Could you check a few things on this drawing? It's one solid part, dimensions in mm from its lowest x, y, z. Coordinates: 2 decimals unless noted, no trailing zeros. Order: outer loops, then holes, each group sorted by start corner. A loop starts at its lowest first (then second) coordinate and runs counter-clockwise, first axis right, second up. Notation, with made-up numbers: M 21,20 L 51,20 A24 cw 51,41 Z; hole C 79,42.5 d8. An arc over 180 degrees is marked long. Write item = value, one per line. Start each with the question number.
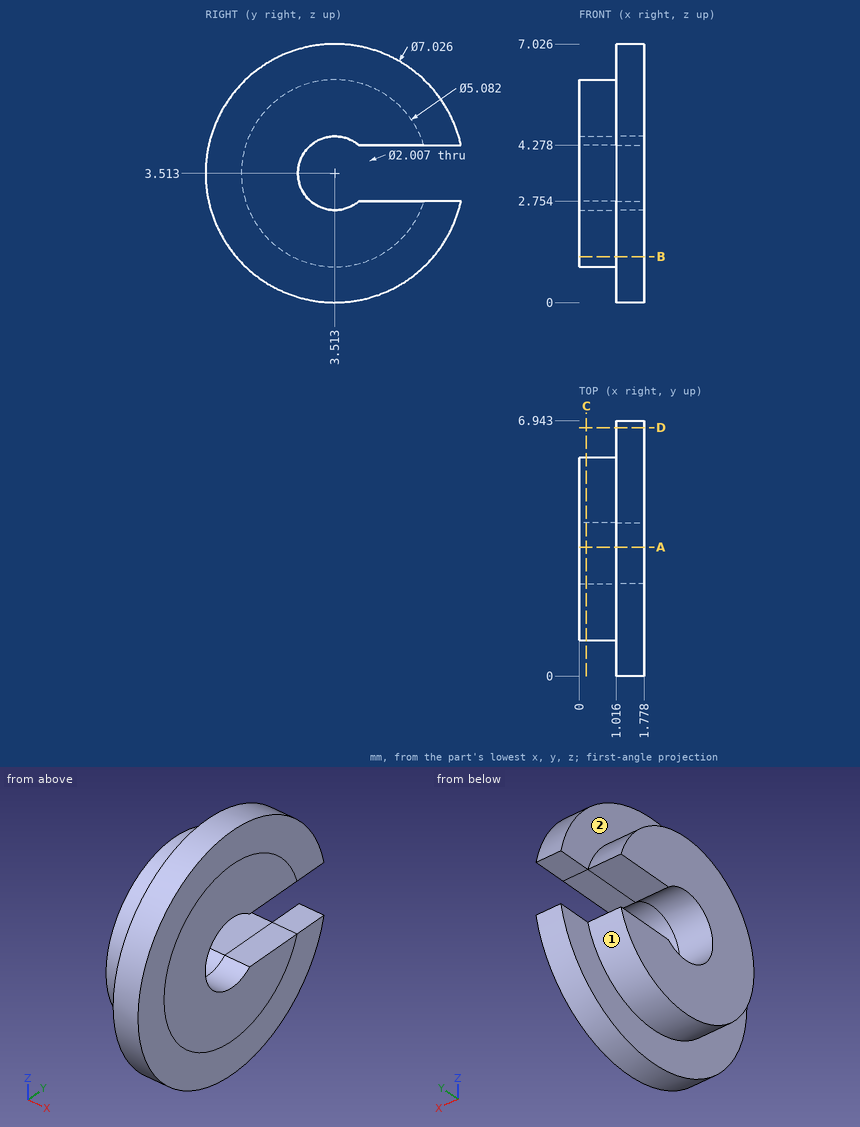
(1) Imagine slicing it at C-C on x = 0.2. List the corners of the cut face in (y, z) for me, plus the area to 3 significant figures.
(2) Thinking about a two-plate mould opening in Y: for the marked faces 1 and 2, which applies, released by +Y, released by -Y, zero draft, split by the parting line, or undercut?
(3) Please list where these lines run through material, in increasing order: probe 1 along X at (y, z) = (0.5, 4); probe 2 along Z at (x, y) = (1.6, 3.5); probe 3 along Y at (x, z) = (1.6, 3.5). Write a range as from..to.
(4) Imagine slicing it at D-D on y = 6.75. List the corners of the cut face in (x, z) for me.
(5) Will these pins go through, and if not, where does the flat tip stop? P1, Ø0.5, axis at x = 0.5, y = 5, coming from the -Z side; P2, Ø3.5, axis at y = 4.5, z = 4, coming from the -X side; P3, Ø0.6, axis at x = 1.5, y = 6.5, coming from the +Z side (1 decimal); P4, Ø0.8, axis at x = 1.5, y = 6.5, coming from the -Z side (1 decimal).
(6) Imagine slicing it at B-B on z = 1.25. List the corners of the cut face in (x, y) for me.
(7) Imagine slicing it at A-A on y = 3.5. List the corners of the cut face in (x, z) for me (1 decimal).
Response:
q1.outline = M 4.16,4.28 L 5.94,4.28 A2.54 ccw long 5.94,2.75 L 4.17,2.75 A1 cw long Z
q1.area = 14.7 mm2
q2.face_1 = split by the parting line
q2.face_2 = zero draft
q3.probe_1 = 1.02..1.78
q3.probe_2 = 0..2.51, 4.52..7.03
q3.probe_3 = 0..2.51
q4.outline = M 1.02,2.15 L 1.78,2.15 L 1.78,2.75 L 1.02,2.75 Z; M 1.02,4.28 L 1.78,4.28 L 1.78,4.88 L 1.02,4.88 Z
q5.P1 = 1.29
q5.P2 = 0
q5.P3 = 5.8
q5.P4 = 1.1
q6.outline = M 0,2.36 L 1.02,2.36 L 1.02,0.83 L 1.78,0.83 L 1.78,6.2 L 1.02,6.2 L 1.02,4.67 L 0,4.67 Z
q7.outline = M 0,1 L 1,1 L 1,0 L 1.8,0 L 1.8,2.5 L 0,2.5 Z; M 0,4.5 L 1.8,4.5 L 1.8,7 L 1,7 L 1,6.1 L 0,6.1 Z
